Geometry: final body of the model. Coordinates: model frame, mm. A direction names the side the tool comes from. Round coordinates to 2 decimals unless told otherwise and drop trailing zeros. Loops run counter-clockwise (first coordinate to the right, second up) from the corner with the lowest first, then second, coordinate; pieces in that order, holes last. Notation, with made-up numbers: M 12,84 L 34,84 A17 cw 34,101 Z; hole C -26,36 d11. An arc over 180 degrees is marked long. Write each question's results on one line, items separated by ' | '.
Autodesk Inventor part; units mm, degrees
ref_plane "YZ Plane" through (0, 0, 0) normal (1, 0, 0) x (0, 1, 0)
ref_plane "XZ Plane" through (0, 0, 0) normal (0, 1, 0) x (-1, 0, 0)
ref_plane "XY Plane" through (0, 0, 0) normal (0, 0, 1) x (1, 0, 0)
sketch "Sketch1" plane through (0, 0, 0) normal (0, 0, 1) x (1, 0, 0)
  circle A0 centre (0, 0) radius 22.5
  dimension "d0" = 45
extrude "Extrusion1" add sketch "Sketch1" along normal blind 20
sketch "Sketch2" plane through (0, 0, 20) normal (0, 0, 1) x (1, 0, 0)
  circle A0 centre (0, 0) radius 17.5
  dimension "d3" = 35
extrude "Extrusion2" add sketch "Sketch2" along normal blind 10
chamfer "Chamfer1" distance 1 angle 45 1 edges at (-17.5, 0, 20)
chamfer "Chamfer2" distance 1 angle 45 1 edges at (-17.5, 0, 30)
chamfer "Chamfer3" distance 1 angle 45 1 edges at (-22.5, 0, 0)
sketch "Sketch3" plane through (0, 0, 30) normal (0, 0, 1) x (1, 0, 0)
  circle A0 centre (0, 0) radius 5
  dimension "d15" = 10
extrude "Extrusion3" cut sketch "Sketch3" against normal blind 3.2
1. Access query for faces 4 (the face through (0, 0, 0)), 5 (the face through (-13.887, 10.648, 24.944)). Directions: +Z, -Z, +X, -X, +Y, -Y. A direction counts if a zero-diameter tool reaches every point of the face in a straight line with its end or side. Return the directions, or none.
Answer key:
face 4: -Z, +X, -X, +Y, -Y | face 5: +Z
2. Section A-A (y = 0). Output: boundary loops of the cut face in (x, z).
Answer key:
outline: M -22.5,1 L -21.5,0 L 21.5,0 L 22.5,1 L 22.5,20 L 18.5,20 L 17.5,21 L 17.5,29 L 16.5,30 L 5,30 L 5,26.8 L -5,26.8 L -5,30 L -16.5,30 L -17.5,29 L -17.5,21 L -18.5,20 L -22.5,20 Z
3. Section D-D (z = 24.75). Output: boundary loops of the cut face in (x, y).
Answer key:
outline: C 0,0 d35
4. Draft query along Y for faces 1 (the face through (10.382, 19.961, 10.367)), 2 (the face through (-5, -18, 20)), 3 (the face through (0, 0, 26.8)). Return one class per face: pulls with the +Y half, pulls with the -Y half, needs draft (parallel to the pull), parting line crosses it, or undercut.
Answer key:
face 1: parting line crosses it | face 2: needs draft | face 3: undercut
5. Ray query, probe 1 along Y at (x, z) = (0, 27.6); probe 2 along Z at (x, y) = (13, 15.5); probe 3 along Y at (x, z) = (0, 29.1). Return the intervals inside material, ascending.
Answer key:
probe 1: y = -17.5 to -5, 5 to 17.5 | probe 2: z = 0 to 20 | probe 3: y = -17.4 to -5, 5 to 17.4
6. Section C-C (z = 11.75). Output: boundary loops of the cut face in (x, y).
Answer key:
outline: C 0,0 d45
7. Pin query (flat end, axial travel): P1, Ø4, axis at x = 10, z = 10, coming from the -Y side; P2, Ø3, axis at y = -18, z = 18.5, coming from the +X side; P3, Ø4, axis at x = -7.5, z = 7, coming from the -Y side; P4, Ø13.5, axis at x = 3.5, y = 2, coming from the +Z side. Return the tip coordinate at first contact, or that it passes through.
Answer key:
P1: stops at y = -21.03 | P2: stops at x = 15.3 | P3: stops at y = -21.82 | P4: stops at z = 30
